Work out the finished part from the listing and answer in its coordinate system (mm). A direction names the side the tool comes from. Give positions to 0.01 mm unless a question says otherwise; leave off trailing zeros. Loops run counter-clockwise (first coordinate to the right, second up) from the corner with the lowest first, then second, coordinate; pieces in that order, holes last. Notation, with made-up numbers: M 67,10 L 82,10 A29 cw 82,41 Z; hole C -20,86 d4. An arc over 180 degrees is marked long. Write item = value, one per line. Start each with the question number.
1. Section B-B on z = 0 is taken. Determine the outline of the cut face in (x, y) (3 decimals).
2. Section D-D on y = 8.5 is taken. Determine the outline of the cut face in (x, z) (3 decimals), plus the area to 3 significant figures.
3. Section C-C on y = 21.5 is taken. Determine the outline of the cut face in (x, z) (3 decimals), plus the area to 3 significant figures.
4. Section A-A on x = 0 is taken. Determine the outline of the cut face in (y, z) (3 decimals), plus the area to 3 significant figures.
5. Flat-ended cylindrical pins translate along their axes: pin 1 Ø2.5 at (x, z) = (0.5, 0) entering from +Y; pin 2 Ø1.5 at (x, y) = (5, 11) entering from +Z; pin 3 Ø5 at (y, z) = (9, -6.5) entering from +X. Find the tip coordinate at first contact, or state that the pin passes through.
6. For faces 1 (the face through (-2, 25, 2)), 2 (the face through (-2.44, 3.45, -0.54)), 3 (the face through (-2.44, 21.45, -0.54)), determine the directions among +Z, -Z, +X, -X, +Y, -Y from which every point of the face is accessible in a straight line to the end or side of a thin tool.
7. Consider L1, parallel to X at y = 19.5, z = 0 (3 decimals); L2, parallel to Z at x = 2, y = 4.5; L3, parallel to Z at x = -2.25, y = 20.25. Determine where each line is inside the solid, lowest interval first. Write a range as [from, to].
```python
from build123d import *

# Parameters (mm, degrees)
SKETCH1_R           = 9.455
SKETCH1_R_2         = 2.5
BOSS_EXTRUDE1_DEPTH = 25
BOSS_EXTRUDE2_START = -18
SKETCH2_R           = 2.5
BOSS_EXTRUDE2_DEPTH = 11


with BuildPart() as part:
    # Sketch1 → Boss-Extrude1 (new body)
    with BuildSketch(Plane(origin=(0, 0, 0), x_dir=(1, 0, 0), z_dir=(0, 1, 0))):
        with Locations(Location((0, 0, 0), (0, 0, 270))):
            Circle(SKETCH1_R)
        with Locations(Location((0, 0, 0), (0, 0, 270))):
            Circle(SKETCH1_R_2, mode=Mode.SUBTRACT)
    extrude(amount=BOSS_EXTRUDE1_DEPTH)

    # Sketch2 → Boss-Extrude2 (add)
    with BuildSketch(Plane(origin=(0, 25, 0), x_dir=(1, 0, 0), z_dir=(0, 1, 0)).offset(BOSS_EXTRUDE2_START)):
        with Locations(Location((0, 0, 0), (0, 0, 270))):
            Circle(SKETCH2_R)
    extrude(amount=BOSS_EXTRUDE2_DEPTH)


solid = part.part
```
Verdict:
q1.outline = M -9.455,0 L -2.5,0 L -2.5,7 L 2.5,7 L 2.5,0 L 9.455,0 L 9.455,25 L 2.5,25 L 2.5,18 L -2.5,18 L -2.5,25 L -9.455,25 Z
q2.outline = C 0,0 d18.91
q2.area = 281 mm2
q3.outline = C 0,0 d18.91; hole C 0,0 d5
q3.area = 261 mm2
q4.outline = M 0,-9.455 L 25,-9.455 L 25,-2.5 L 18,-2.5 L 18,2.5 L 25,2.5 L 25,9.455 L 0,9.455 L 0,2.5 L 7,2.5 L 7,-2.5 L 0,-2.5 Z
q4.area = 403 mm2
q5.pin_1 = 18
q5.pin_2 = 8.45
q5.pin_3 = 8.57
q6.face_1 = +Z, -Z, +X, -X, +Y
q6.face_2 = -Y
q6.face_3 = +Y
q7.L1 = [-9.455, -2.5], [2.5, 9.455]
q7.L2 = [-9.24, -1.5], [1.5, 9.24]
q7.L3 = [-9.18, -1.09], [1.09, 9.18]
